Could you check a few things on this model? Use its own coordinates, in mm. A direction names the side the tool comes from. Coordinates: 2 decimals unless noted, no trailing zeros. Order: outer loops, then holes, each group sorted by start corner. A loop starts at its lowest first (then second) coordinate and runs counter-clockwise, first axis right, second up. Notation, with made-up numbers: (-32, 44) - (-28, 44) arc R16 ccw to (-28, 65) - close; hole circle Ø9 at (-17, 34). An arc over 180 degrees is marked (long way). Answer as a JSON object with one key per item and string values. Group by question number.
(1) Imagine slicing it at D-D, the plane z = 16. Write out the boundary of the cut face in (x, y), and give its area (3 significant figures).
(2) Imagine slicing it at A-A, the plane z = -20. Write out the boundary of the cut face in (x, y), and give its area (3 significant figures).
(3) Will these pins go through, and if not, where does the flat tip stop? P1, Ø5, axis at x = 4.5, y = 54, coming from the +Z side; P2, Ø0.8, axis at x = 6, y = -30.5, coming from the -Z side; P3, Ø2, axis at x = 11, y = -51.5, coming from the +Z side; P4, Ø1, axis at y = 20, z = 9.5, coming from the +X side.
(4) Imagine slicing it at C-C, the plane x = 1.5. Give the number of separate pieces and of enclosed holes in the cut face, and give its area (3 significant figures).
(5) Please list where these lines run through material, in increasing order: probe 1 along Z at (x, y) = (0.25, 28); probe 2 along Y at (x, z) = (11.25, -26.5); probe 3 along X at (y, z) = (5, -3.5).
(6) We'd pull the mould along Z, two halves only. Please class faces 1 (the flat face through (8.874, 2.846, -11.978)), 2 (the flat face through (8.944, -34.673, -13.959)), 3 (the flat face through (8.874, -1.883, -28.77)): pulls with the +Z half, pulls with the -Z half, needs draft (parallel to the pull), parting line crosses it, or undercut.
(7) Which directions (+Z, -Z, +X, -X, +Y, -Y) give clear straight access to the entire face, cutting with the end or side of a thin tool? Please do faces 4 (the flat face through (1.48, 35.13, 9.06)), 5 (the flat face through (16.521, 38.275, 0.664)), 6 (the flat face through (9.08, -24.85, -11.08)), 7 (the flat face through (9.13, -28.82, -26.77)), 8 (the flat face through (9, -51, -13.8)).
(8) Imagine slicing it at B-B, the plane y = 36. Write out the boundary of the cut face in (x, z).
from build123d import *

# Parameters (mm, degrees)
BOSS_EXTRUDE1_DEPTH = 18
CUT_EXTRUDE1_DEPTH  = 18
BOSS_EXTRUDE2_DEPTH = 18
LPATTERN1_COUNT     = 5
LPATTERN1_PITCH     = 5
FILLET1_R           = 8
FILLET2_R           = 5
SKETCH4_R           = 1.5
CUT_EXTRUDE2_DEPTH  = 18
CUT_EXTRUDE3_DEPTH  = 6
SKETCH6_R           = 1.75
BOSS_EXTRUDE3_DEPTH = 1.5
SKETCH7_R           = 1.75
BOSS_EXTRUDE4_DEPTH = 1.5
CUT_EXTRUDE4_DEPTH  = 3


with BuildPart() as part:
    # Sketch1 → Boss-Extrude1 (new body)
    with BuildSketch(Plane(origin=(0, 0, 0), x_dir=(0, 0, -1), z_dir=(1, 0, 0))):
        with BuildLine():
            Line((24.799627928, -4.804973216), (32.853416759, 1.122630471))
            ThreePointArc((32.853416759, 1.122630471), (35.038056902, 9.373242879), (26.787444494, 11.557883023))
            Line((26.787444494, 11.557883023), (13.901382366, 2.073717122))
            Line((13.901382366, 2.073717122), (10, 3.639702343))
            Line((10, 3.639702343), (0, 0))
            Line((0, 0), (-5, -1.819851171))
            Line((-5, -1.819851171), (-5, -11.819851171))
            Line((-5, -11.819851171), (8, -17.804973216))
            Line((8, -17.804973216), (13.799627928, -47.804973216))
            Line((13.799627928, -47.804973216), (13.799627928, -54.804973216))
            Line((13.799627928, -54.804973216), (24.799627928, -54.804973216))
            Line((24.799627928, -54.804973216), (24.799627928, -4.804973216))
        make_face()
        Polygon((10, 3.639702343), (0, 0), (-25.477916399, 70), (-1.477916399, 74.639702343), align=None)
    extrude(amount=BOSS_EXTRUDE1_DEPTH)

    # Sketch2 → Cut-Extrude1 (cut)
    with BuildSketch(Plane(origin=(18, 0, 0), x_dir=(0, 0, -1), z_dir=(1, 0, 0))):
        Polygon((12.09390479, -22.804973216), (22.09390479, -22.804973216), (22.09390479, -47.804973216), align=None)
    extrude(amount=-CUT_EXTRUDE1_DEPTH, mode=Mode.SUBTRACT)

    # Sketch3 → Boss-Extrude2 (add)
    with BuildSketch(Plane(origin=(18, 0, 0), x_dir=(0, 0, -1), z_dir=(1, 0, 0))):
        Polygon((24.799627928, -47.804973216), (24.799627928, -49.804973216), (28.799627928, -47.804973216), align=None)
        Polygon((24.799627928, -47.804973216), (28.799627928, -47.804973216), (24.799627928, -45.804973216), align=None)
    boss_extrude2 = extrude(amount=-BOSS_EXTRUDE2_DEPTH)

    # LPattern1: Boss-Extrude2 ×5
    with Locations(*[(0, i * LPATTERN1_PITCH, 0) for i in range(1, LPATTERN1_COUNT)]):
        add(boss_extrude2)

    # Fillet1
    # the kernel refuses this fillet: 8 mm, written as the material it takes off along each edge
    with BuildSketch(Plane(origin=(-13.990868289, -1.819851171, 5), x_dir=(0, 0.34202014332566644, -0.9396926207859092), z_dir=(1, 0, 0))) as fillet1_piece_1:
        with BuildLine():
            CenterArc((5.603477455, -7.995007423), FILLET1_R, 92.024312837, 67.975687163)
            Line((-1.914063511, -5.258846276), (-2.06441433, -5.204123053))
            Line((-2.06441433, -5.204123053), (-0.150350819, 0.054723223))
            Line((-0.150350819, 0.054723223), (0, 0.16))
            ThreePointArc((0, 0.16), (2.660444431, 0.16), (5.315237091, 0.159900148))
            Line((5.315237091, 0.159900148), (5.320888862, 0))
        make_face()
    extrude(amount=45.981736579, mode=Mode.SUBTRACT)
    with BuildSketch(Plane(origin=(-12.809954869, -11.819851171, 5), x_dir=(0, 1, 0), z_dir=(1, 0, 0))) as fillet1_piece_2:
        with BuildLine():
            CenterArc((FILLET1_R * 0.640497743455, -FILLET1_R), FILLET1_R, 90, 65.278940391)
            Line((-FILLET1_R * 0.267856781688, -FILLET1_R * 0.581799023611), (-FILLET1_R * 0.286023872191, -FILLET1_R * 0.573435004083))
            Line((-FILLET1_R * 0.286023872191, -FILLET1_R * 0.573435004083), (-FILLET1_R * 0.0128099548691, FILLET1_R * 0.02))
            Line((-FILLET1_R * 0.0128099548691, FILLET1_R * 0.02), (FILLET1_R * 0.640497743455, FILLET1_R * 0.02))
            Line((FILLET1_R * 0.640497743455, FILLET1_R * 0.02), (FILLET1_R * 0.640497743455, 0))
        make_face()
    extrude(amount=43.619909738, mode=Mode.SUBTRACT)

    # Fillet2
    fillet2_edges = [part.edges().sort_by_distance(p)[0] for p in [
        (9, 70, 25.477916399),
        (9, 74.639702343, 1.477916399),
    ]]
    fillet(fillet2_edges, radius=FILLET2_R)

    # Sketch4 → Cut-Extrude2 (cut)
    with BuildSketch(Plane(origin=(18, 0, 0), x_dir=(0, 0, -1), z_dir=(1, 0, 0))):
        with Locations((-18.775111552, 66.203217038)):
            Circle(SKETCH4_R)
    extrude(amount=-CUT_EXTRUDE2_DEPTH, mode=Mode.SUBTRACT)

    # Sketch5 → Cut-Extrude3 (cut)
    with BuildSketch(Plane(origin=(0, 0.849397963, -4.393719597), x_dir=(1, 0, 0), z_dir=(0, -0.1898066444194718, 0.981821489749649))):
        Polygon((15, -26.499758484), (9, -26.499758484), (3, -26.499758484), (5, -36.691893202), (9, -36.691893202), (13, -36.691893202), align=None)
    extrude(amount=-CUT_EXTRUDE3_DEPTH, mode=Mode.SUBTRACT)

    # Sketch6 → Boss-Extrude3 (add)
    with BuildSketch(Plane(origin=(18, 0, 0), x_dir=(0, 0, -1), z_dir=(1, 0, 0))):
        with Locations((29.820430626, 6.340256747)):
            Circle(SKETCH6_R)
    boss_extrude3 = extrude(amount=BOSS_EXTRUDE3_DEPTH)

    # Sketch7 → Boss-Extrude4 (add)
    with BuildSketch(Plane(origin=(18, 0, 0), x_dir=(0, 0, -1), z_dir=(1, 0, 0))):
        with Locations((3, -6.695869224)):
            Circle(SKETCH7_R)
    boss_extrude4 = extrude(amount=BOSS_EXTRUDE4_DEPTH)

    # Sketch8 → Cut-Extrude4 (cut)
    with BuildSketch(Plane(origin=(18, 0, 0), x_dir=(0, 0, -1), z_dir=(1, 0, 0))):
        with BuildLine():
            Line((-17.332707084, 61.238673153), (-5.781480677, 63.471766995))
            ThreePointArc((-5.781480677, 63.471766995), (-5.018988164, 63.309720411), (-4.604490469, 62.649534384))
            Line((-4.604490469, 62.649534384), (3.388275701, 13.207947746))
            ThreePointArc((3.388275701, 13.207947746), (3.349595335, 12.731591312), (3.094265813, 12.327588269))
            Line((3.094265813, 12.327588269), (1.345046537, 10.645343239))
            ThreePointArc((1.345046537, 10.645343239), (0.425917391, 10.391976204), (-0.28781976, 11.024093693))
            Line((-0.28781976, 11.024093693), (-18.08259306, 59.914831519))
            ThreePointArc((-18.08259306, 59.914831519), (-18.013004637, 60.74971948), (-17.332707084, 61.238673153))
        make_face()
    cut_extrude4 = extrude(amount=-CUT_EXTRUDE4_DEPTH, mode=Mode.SUBTRACT)

    # Mirror1: Boss-Extrude3, Boss-Extrude4, Cut-Extrude4 across plane
    add(boss_extrude3.mirror(Plane(origin=(9, 0, 0), x_dir=(0, 0, 1), z_dir=(1, 0, 0))))
    add(boss_extrude4.mirror(Plane(origin=(9, 0, 0), x_dir=(0, 0, 1), z_dir=(1, 0, 0))))
    add(cut_extrude4.mirror(Plane(origin=(9, 0, 0), x_dir=(0, 0, 1), z_dir=(1, 0, 0))), mode=Mode.SUBTRACT)


solid = part.part
Result set:
{
 "1": {"outline": "(0, 43.96) - (18, 43.96) - (18, 54.19) - (15, 54.19) - (15, 61.5) - (18, 61.5) - (18, 71.83) - (0, 71.83) - (0, 61.5) - (3, 61.5) - (3, 54.19) - (0, 54.19) - close", "area": "458 mm^2"},
 "2": {"outline": "(0, -54.8) - (18, -54.8) - (18, -42.57) - (0, -42.57) - close; (0, -22.8) - (18, -22.8) - (18, 6.56) - (0, 6.56) - close", "area": "749 mm^2"},
 "3": {"P1": "stops at z = 20.56", "P2": "stops at z = -24.99", "P3": "stops at z = -13.8", "P4": "passes through"},
 "4": {"separate pieces": "1", "enclosed holes": "3", "area": "1,900 mm^2"},
 "5": {"probe 1": "z = -6.06 to -1, 6.47 to 10.19", "probe 2": "y = -48.95 to -46.66, -43.95 to -41.66, -38.95 to -36.66, -33.95 to -31.66, -28.95 to -26.66, -3.55 to 11.35", "probe 3": "x = 0 to 18"},
 "6": {"face 1": "undercut", "face 2": "pulls with the +Z half", "face 3": "pulls with the -Z half"},
 "7": {"face 4": "-X", "face 5": "+X", "face 6": "none", "face 7": "-Z, +X, -X", "face 8": "+Z, +X, -X, -Y"},
 "8": {"outline": "(0, -4.77) - (18, -4.77) - (18, 0.3) - (15, 0.3) - (15, 9.38) - (18, 9.38) - (18, 13.1) - (0, 13.1) - (0, 9.38) - (3, 9.38) - (3, 0.3) - (0, 0.3) - close"}
}
